Work out the finished part from the listing and answer in its coordinate system (mm). A direction names the side the tool comes from. Give positions to 0.01 mm unless a question says otherwise; leave off trailing zeros. Loops run counter-clockwise (first coordinate to the right, second up) from the corner with the lowest first, then second, coordinate; pieces in that order, holes last.
```python
from build123d import *

# Parameters (mm, degrees)
F1_DEPTH = 11
F2_W     = 25
F2_H     = 17
F3_DEPTH = 2


with BuildPart() as f1:
    # F0 (on Front) → F1 (new body)
    with BuildSketch(Plane.XZ):
        with BuildLine():
            Line((0, 14.117118), (0, 0))
            Line((0, 0), (25, 0))
            Line((25, 0), (25, 14.117118))
            ThreePointArc((25, 14.117118), (23.98797, 19.044242), (21.115752, 23.173542))
            ThreePointArc((21.115752, 23.173542), (20.161384, 23.785734), (19.047972, 24))
            Line((19.047972, 24), (18.98802, 24))
            ThreePointArc((18.98802, 24), (18.037353, 23.310214), (18.3982, 22.192465))
            ThreePointArc((18.3982, 22.192465), (12.5, 4.117118), (6.6018, 22.192465))
            ThreePointArc((6.6018, 22.192465), (6.962647, 23.310214), (6.01198, 24))
            Line((6.01198, 24), (5.952028, 24))
            ThreePointArc((5.952028, 24), (4.838616, 23.785734), (3.884248, 23.173542))
            ThreePointArc((3.884248, 23.173542), (1.01203, 19.044242), (0, 14.117118))
        make_face()
    extrude(amount=F1_DEPTH)

    # F2 (on face) → F3 (join)
    with BuildSketch(Plane(origin=(0, 0, 0), x_dir=(1, 0, 0), z_dir=(0, 0, -1))):
        with Locations((12.5, 5.5)):
            Rectangle(F2_W, F2_H)
    extrude(amount=F3_DEPTH)


solid = f1.part
```
Q1. Consider line 1 along X through (y, z) = (-4, 14); line 2 along Z through (x, y) = (12.5, -7); line 3 along Z through (x, y) = (7.25, -11.25). Determine where each line is inside the solid, lowest interval first.
Q2. Given pin 1 (6 mm diameter, centred on x = 21.5, z = 10.5, fed in from +Y); pin 2 (3.5 mm diameter, centred on x = 16.5, y = 2, fed in from +Z); pin 3 (8 mm diameter, centred on x = 13.5, y = -10.5, fed in from +Z), each flat-ended and moving along its own axis, determine where each tip first touches the part or whether it passes through.
Q3. Section B-B on x = 12.5 is taken. Give the vertices of the cut face in (y, z), plus the area to 3 significant figures.
Q4. Section D-D on z = 8.25 is taken. Give the vertices of the cut face in (x, y).
Q5. Which of the six approach directions +Z, -Z, +X, -X, +Y, -Y give full straight-line access (tool end or side, diameter ignored) to faces 5 (the face through (15, -11, 4)), 6 (the face through (24.016, -5.423, 18.979)), 7 (the face through (15, 0, 4)), 8 (the face through (6.97, -5.42, 23.29))?
Q6. Section C-C on y = -12 is taken. Give the vertices of the cut face in (x, z), plus the area to 3 significant figures.
Q7. Determine the mould class of faces 1 (the face through (12, -13, 0)), 2 (the face through (18.043, -5.423, 23.327)), 3 (the face through (12.851, -5.423, 4.123)), 4 (the face through (12, -14, -1)) for opening direction Z: +Z half, -Z half, draft (parallel to the pull), parting line (faces both ways), or undercut.
Q8. Section A-A on z = 16.75 is taken. Give the vertices of the cut face in (x, y).
Check result:
1. line 1: x = 0 to 2.5, 22.5 to 25
1. line 2: z = -2 to 4.12
1. line 3: z = -2 to 0
2. pin 1: stops at y = 0
2. pin 2: stops at z = 0
2. pin 3: stops at z = 5.46
3. outline: (-14, -2) - (3, -2) - (3, 0) - (0, 0) - (0, 4.12) - (-11, 4.12) - (-11, 0) - (-14, 0) - close
3. area: 79.3 mm2
4. outline: (0, -11) - (4.4, -11) - (4.4, 0) - (0, 0) - close; (20.6, -11) - (25, -11) - (25, 0) - (20.6, 0) - close
5. face 5: +Z, +X, -X, -Y
5. face 6: +Z, +X, +Y, -Y
5. face 7: +Z, +X, -X, +Y
5. face 8: +Y, -Y
6. outline: (0, -2) - (25, -2) - (25, 0) - (0, 0) - close
6. area: 50.0 mm2
7. face 1: +Z half
7. face 2: undercut
7. face 3: undercut
7. face 4: draft
8. outline: (0.28, -11) - (2.85, -11) - (2.85, 0) - (0.28, 0) - close; (22.15, -11) - (24.72, -11) - (24.72, 0) - (22.15, 0) - close
